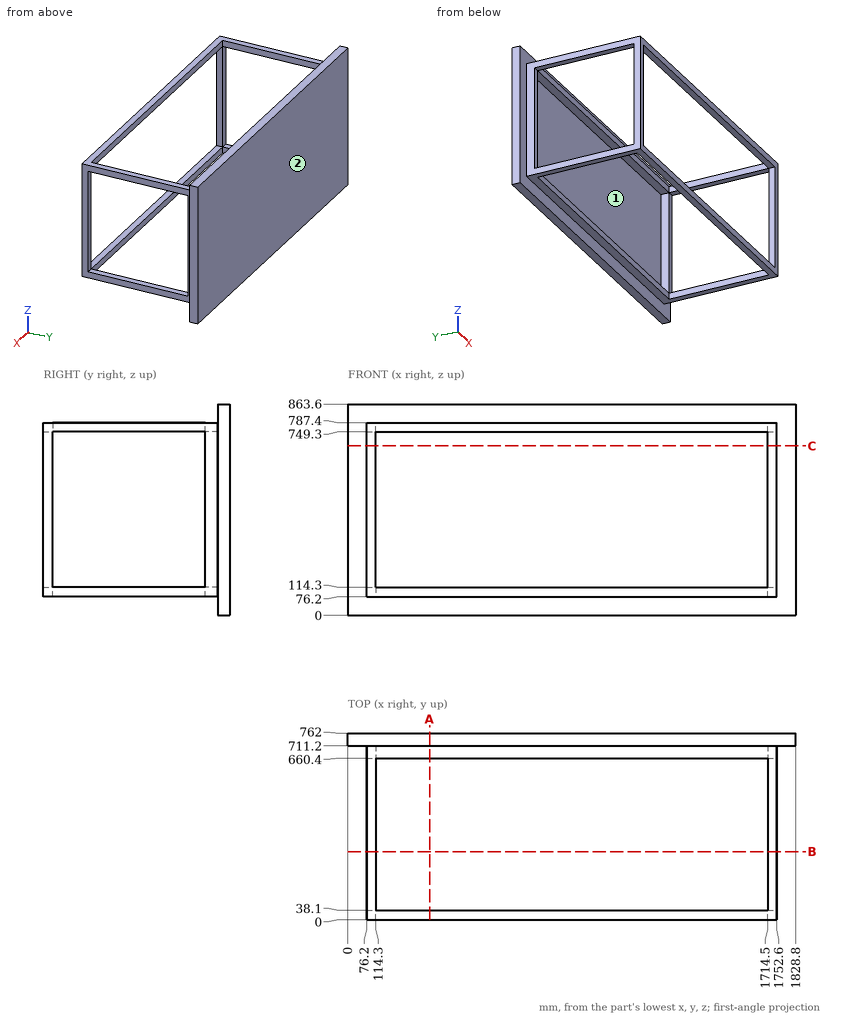
Check sheet for the drawn part. Datum: minimum x, y, z corner. Units: mm. Round coordinates to 2 decimals unless told otherwise and drop trailing zeros. Loops run counter-clockwise (first coordinate to the right, second up) from the corner with the lowest first, then second, coordinate; pieces in that order, holes last. Notation, with made-up numbers: (3.25, -0.5) - (38.25, -0.5) arc R32 cw to (38.25, 32.5) - close; hole circle Ø4 at (84, 89). An arc over 180 degrees is marked (long way). Answer as a JSON object with one key per item and string values. Group by question number.
Q1. Gauge pin test, flat ends, axial feed: P1, Ø11.5, axis at x = 100, y = 321.5, coming from the +Z side; P2, Ø1, axis at x = 1432, z = 128.5, coming from the -Y side; P3, Ø1.5, axis at y = 656, z = 775, coming from the -X side. Record the tip position at first contact, or that the pin passes through.
Q2. Sectioned sample at B-B, the plane y = 278.5. Enter the section's corners in (x, z).
Q3. Scan lines: line 1 along X through (y, z) = (697.5, 173.5); line 2 along Y through (x, z) = (1656.5, 105.5); line 3 along Y through (x, z) = (964, 218). Record each from-to range of solid material in increasing order. Write a range as [from, to].
Q4. Sectioned sample at A-A, the plane x = 334. Enter the section's corners in (y, z), plus the area to 3 significant figures.
Q5. Sectioned sample at C-C, the plane z = 692. Enter the section's corners in (x, y), plus the area to 3 significant figures.
Q6. Mould release check, pull along X, two halves, no side actions. Record for the marked faces 1 and 2: released by +X, released by -X, zero draft, split by the parting line, or undercut.
Solution:
{
 "1": {"P1": "stops at z = 787.4", "P2": "stops at y = 711.2", "P3": "stops at x = 76.2"},
 "2": {"outline": "(76.2, 76.2) - (114.3, 76.2) - (114.3, 114.3) - (76.2, 114.3) - close; (76.2, 749.3) - (114.3, 749.3) - (114.3, 787.4) - (76.2, 787.4) - close; (1714.5, 76.2) - (1752.6, 76.2) - (1752.6, 114.3) - (1714.5, 114.3) - close; (1714.5, 749.3) - (1752.6, 749.3) - (1752.6, 787.4) - (1714.5, 787.4) - close"},
 "3": {"line 1": "x = [76.2, 114.3], [1714.5, 1752.6]", "line 2": "y = [0, 38.1], [660.4, 762]", "line 3": "y = [711.2, 762]"},
 "4": {"outline": "(0, 76.2) - (38.1, 76.2) - (38.1, 114.3) - (0, 114.3) - close; (0, 749.3) - (38.1, 749.3) - (38.1, 787.4) - (0, 787.4) - close; (660.4, 76.2) - (711.2, 76.2) - (711.2, 0) - (762, 0) - (762, 863.6) - (711.2, 863.6) - (711.2, 787.4) - (660.4, 787.4) - (660.4, 749.3) - (711.2, 749.3) - (711.2, 114.3) - (660.4, 114.3) - close", "area": "50,600 mm²"},
 "5": {"outline": "(0, 711.2) - (76.2, 711.2) - (76.2, 660.4) - (114.3, 660.4) - (114.3, 711.2) - (1714.5, 711.2) - (1714.5, 660.4) - (1752.6, 660.4) - (1752.6, 711.2) - (1828.8, 711.2) - (1828.8, 762) - (0, 762) - close; (76.2, 0) - (114.3, 0) - (114.3, 38.1) - (76.2, 38.1) - close; (1714.5, 0) - (1752.6, 0) - (1752.6, 38.1) - (1714.5, 38.1) - close", "area": "99,700 mm²"},
 "6": {"face 1": "undercut", "face 2": "zero draft"}
}
